```python
from build123d import *

# Parameters (mm, degrees)
BOSS_EXTRUDE1_DEPTH = 10.3
SKETCH2_R           = 5.25
BOSS_EXTRUDE2_DEPTH = 1.3
SKETCH3_R           = 3.75
BOSS_EXTRUDE3_DEPTH = 0.7
SKETCH4_R           = 2.75
SKETCH4_R_2         = 1.25
BOSS_EXTRUDE4_DEPTH = 9.4
FILLET1_R           = 1
SKETCH5_R           = 4.3
SKETCH5_R_2         = 2.75
BOSS_EXTRUDE5_DEPTH = 4


with BuildPart() as part:
    # Sketch1 → Boss-Extrude1 (new body)
    with BuildSketch(Plane.XY):
        with BuildLine():
            Line((-3.012059096, 4.3), (-19, 4.3))
            Line((-19, 4.3), (-19, -4.3))
            Line((-19, -4.3), (-3.012059096, -4.3))
            ThreePointArc((-3.012059096, -4.3), (5.25, 0), (-3.012059096, 4.3))
        make_face()
    extrude(amount=BOSS_EXTRUDE1_DEPTH)

    # Sketch2 → Boss-Extrude2 (add)
    with BuildSketch(Plane.XY.offset(10.3)):
        Circle(SKETCH2_R)
    extrude(amount=BOSS_EXTRUDE2_DEPTH)

    # Sketch3 → Boss-Extrude3 (add)
    with BuildSketch(Plane.XY.offset(11.6)):
        Circle(SKETCH3_R)
    extrude(amount=BOSS_EXTRUDE3_DEPTH)

    # Sketch4 → Boss-Extrude4 (add)
    with BuildSketch(Plane.XY.offset(12.3)):
        Circle(SKETCH4_R)
        Circle(SKETCH4_R_2, mode=Mode.SUBTRACT)
    extrude(amount=BOSS_EXTRUDE4_DEPTH)

    # Fillet1
    fillet1_edges = [part.edges().sort_by_distance(p)[0] for p in [
        (-2.75, 0, 21.7),
    ]]
    fillet(fillet1_edges, radius=FILLET1_R)

    # Sketch5 → Boss-Extrude5 (add)
    with BuildSketch(Plane.ZY.offset(19)):
        with Locations((5.15, 0)):
            Circle(SKETCH5_R)
        with Locations((5.15, 0)):
            Circle(SKETCH5_R_2, mode=Mode.SUBTRACT)
    extrude(amount=BOSS_EXTRUDE5_DEPTH)


solid = part.part
```
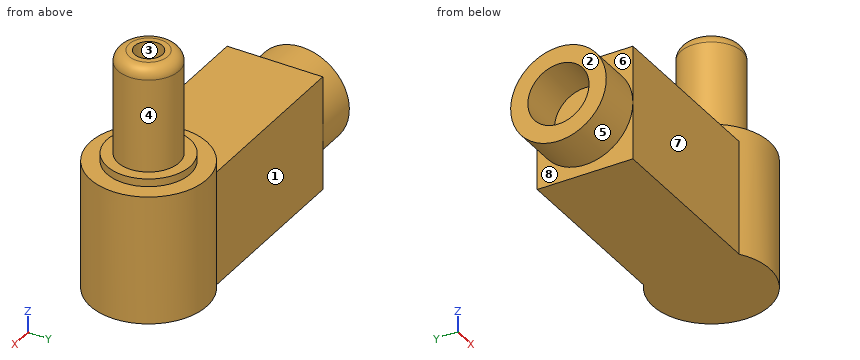
CAD build for the part. Positions are in the model's coordinates, mm. Face numbers are marked on the shaded views. A direction names the side the tool comes from. Coordinates: 2 decimals unless noted, no trailing zeros. Write each loop counter-clockwise with the first axis right and the second up, starting at its lowest first coordinate (ties: lowest second). Pieces come first, ordered by that corner, then holes.
(1) Cut at A-A, the plane z = 18.5. List the corners of the cut face in (x, y).
(2) 3-axis set-ups, long thin cutter, end or side, ignore diameter. For the marked faces 4, 5, 6, 7 and 8: which of +Z, -Z, +X, -X, +Y, -Y reach the whole face in a straight line?
(3) Cut at D-D, the plane z = 10.75. List the corners of the cut face in (x, y), and give its area (3 significant figures).
(4) Drill centre lines: probe 1 along Y at (x, z) = (0, 15); probe 2 along Z at (x, y) = (-4.75, -2); probe 3 along Y at (x, z) = (-20.55, 5.15). Where is each one in solid material? Low to high.
(5) Flat gauge pins, fed straight in: pin 1 (11.5 mm diameter, centred on x = -14, z = 4.5, fed in from +Y); pin 2 (3 mm diameter, centred on x = 0, y = 0, fed in from +Z); pin 3 (2 mm diameter, centred on x = -19, z = 11, fed in from -Y); pin 4 (4 mm diameter, centred on y = -3.5, z = 17, fed in from +X). Where does each tip first touch, or does it go through?
(6) Two-plate mould, pull along X, no slides. Class the marked faces 1, 2 and 3: +X half, -X half, draft (parallel to the pull), parting line (faces both ways), or undercut.
(7) Cut at B-B, the plane z = 4.25. List the corners of the cut face in (x, y), and give its area (3 significant figures).
(8) Cut at C-C, the plane x = -15.5. List the corners of the cut face in (y, z).
Geometry says:
1. outline: circle Ø5.5 at (0, 0); hole circle Ø2.5 at (0, 0)
2. face 4: +Z
2. face 5: -X
2. face 6: +Z, -X
2. face 7: +Z, -Z, -X, -Y
2. face 8: -Z, -X
3. outline: circle Ø10.5 at (0, 0)
3. area: 86.6 mm2
4. probe 1: y = -2.75 to -1.25, 1.25 to 2.75
4. probe 2: z = 0 to 11.6
4. probe 3: y = -4.3 to -2.75, 2.75 to 4.3
5. pin 1: stops at y = 4.3
5. pin 2: stops at z = 21.7
5. pin 3: stops at y = -4.3
5. pin 4: stops at x = 2.3
6. face 1: draft
6. face 2: -X half
6. face 3: undercut
7. outline: (-23, -4.2) - (-19, -4.2) - (-19, -4.3) - (-3.01, -4.3) arc R5.25 ccw (long way) to (-3.01, 4.3) - (-19, 4.3) - (-19, 4.2) - (-23, 4.2) - (-23, 2.6) - (-19, 2.6) - (-19, -2.6) - (-23, -2.6) - close
7. area: 223 mm2
8. outline: (-4.3, 0) - (4.3, 0) - (4.3, 10.3) - (-4.3, 10.3) - close
